```python
from build123d import *

# Parameters (mm, degrees)
SKETCH1_W           = 93.98
SKETCH1_H           = 66.04
SKETCH1_W_2         = 83.82
SKETCH1_H_2         = 55.88
BOSS_EXTRUDE1_DEPTH = 15.24
SKETCH3_W           = 83.82
SKETCH3_H           = 55.88
BOSS_EXTRUDE2_DEPTH = 7.62
BOSS_EXTRUDE3_DEPTH = 10
FILLET1_R           = 2.54
CUT_EXTRUDE1_DEPTH  = 16.24


with BuildPart() as part:
    # Sketch1 → Boss-Extrude1 (new body)
    with BuildSketch(Plane(origin=(0, 0, 0), x_dir=(1, 0, 0), z_dir=(0, 1, 0))):
        Rectangle(SKETCH1_W, SKETCH1_H)
        Rectangle(SKETCH1_W_2, SKETCH1_H_2, mode=Mode.SUBTRACT)
    extrude(amount=BOSS_EXTRUDE1_DEPTH)

    # Sketch3 → Boss-Extrude2 (add)
    with BuildSketch(Plane(origin=(0, 0, 0), x_dir=(1, 0, 0), z_dir=(0, 1, 0))):
        Rectangle(SKETCH3_W, SKETCH3_H)
    extrude(amount=BOSS_EXTRUDE2_DEPTH)

    # Sketch4 → Boss-Extrude3 (add)
    with BuildSketch(Plane.XZ):
        with BuildLine():
            Line((-30.48, 7.62), (30.48, 7.62))
            ThreePointArc((30.48, 7.62), (31.75, 6.35), (30.48, 5.08))
            Line((30.48, 5.08), (-30.48, 5.08))
            ThreePointArc((-30.48, 5.08), (-31.75, 6.35), (-30.48, 7.62))
        make_face()
    extrude(amount=BOSS_EXTRUDE3_DEPTH)

    # Fillet1
    fillet1_edges = [part.edges().sort_by_distance(p)[0] for p in [
        (46.99, 15.24, 0),
        (0, 15.24, -33.02),
        (-46.99, 15.24, 0),
        (0, 0, -33.02),
        (46.99, 0, 0),
        (0, 0, 33.02),
        (-46.99, 0, 0),
        (-46.99, 7.62, -33.02),
        (46.99, 7.62, -33.02),
        (46.99, 7.62, 33.02),
        (-46.99, 7.62, 33.02),
        (0, 15.24, 33.02),
    ]]
    fillet(fillet1_edges, radius=FILLET1_R)

    # Sketch5 → Cut-Extrude1 (cut, through all)
    with BuildSketch(Plane.XZ):
        with BuildLine():
            Line((38.1, 0), (8.720286281, 0))
            add(Edge.make_bspline(
                [(8.720286281, 0), (0.717932636, -10.320966423), (24.690327376, -11.221788079), (14.302617373, -24.27956655), (19.287221421, -25.4)],
                knots=[0, 0, 0, 0, 0.689243554, 1, 1, 1, 1], degree=3))
            Line((19.287221421, -25.4), (38.1, -25.4))
            Line((38.1, -25.4), (38.1, 0))
        make_face()
        with BuildLine():
            add(Edge.make_bspline(
                [(-38.1, -17.337980958), (-35.187970865, -6.837732589), (-22.396079464, -19.547216799), (-11.076568018, -5.424698839), (8.04848315, -15.407822573), (0.32989112, -20.213116903), (-0.131881687, -22.594944987), (-0.12685046, -22.796669294)],
                knots=[0, 0, 0, 0, 0.327916539, 0.565865574, 0.827054789, 0.928649045, 0.941908126, 0.941908126, 0.941908126, 0.941908126], degree=3))
            Line((-38.1, -17.337980958), (-38.1, -25.4))
            Line((-38.1, -25.4), (-2.666060814, -25.4))
            ThreePointArc((-2.666060814, -25.4), (-0.84775666, -24.633519101), (-0.12685046, -22.796669294))
        make_face()
        with BuildLine():
            ThreePointArc((-20.809664595, 23.563761473), (-23.399285475, 24.661043475), (-26.141098135, 24.03444358))
            ThreePointArc((-26.141098135, 24.03444358), (-32.141459521, 16.03667712), (-22.24223462, 14.631703292))
            ThreePointArc((-22.24223462, 14.631703292), (-20.680528135, 15.549204987), (-18.904626197, 15.192962357))
            ThreePointArc((-18.904626197, 15.192962357), (-17.075188661, 14.538079772), (-15.140614659, 14.720113645))
            ThreePointArc((-15.140614659, 14.720113645), (-13.518109108, 14.699820982), (-12.238965098, 13.701458994))
            ThreePointArc((-12.238965098, 13.701458994), (-9.256805246, 11.946815164), (-6.043815629, 13.230851799))
            ThreePointArc((-6.043815629, 13.230851799), (-4.644606266, 14.021459072), (-3.050933479, 13.813965102))
            ThreePointArc((-3.050933479, 13.813965102), (-0.202264641, 13.116417687), (2.681966092, 13.648112737))
            ThreePointArc((2.681966092, 13.648112737), (4.032557322, 13.814175625), (5.275046214, 13.259292838))
            ThreePointArc((5.275046214, 13.259292838), (7.732359851, 12.317746114), (10.257976284, 13.056773974))
            ThreePointArc((10.257976284, 13.056773974), (11.524940775, 13.507829697), (12.844614733, 13.248771918))
            ThreePointArc((12.844614733, 13.248771918), (15.999143067, 12.5855131), (19.076925277, 13.543749992))
            ThreePointArc((19.076925277, 13.543749992), (20.340690392, 13.925639815), (21.625421379, 13.621652327))
            ThreePointArc((21.625421379, 13.621652327), (23.29387293, 13.01462201), (25.066504565, 12.914654647))
            ThreePointArc((25.066504565, 12.914654647), (25.635512485, 12.901960546), (26.187409107, 12.762887643))
            ThreePointArc((26.187409107, 12.762887643), (32.302173237, 15.205977496), (30.433254549, 21.519943868))
            ThreePointArc((30.433254549, 21.519943868), (29.982257618, 21.867122384), (29.619886936, 22.306005788))
            ThreePointArc((29.619886936, 22.306005788), (26.018947716, 24.881341954), (21.625421379, 24.337240894))
            ThreePointArc((21.625421379, 24.337240894), (20.340690392, 24.033253406), (19.076925277, 24.415143229))
            ThreePointArc((19.076925277, 24.415143229), (13.537462145, 25.005428585), (9.633287177, 21.031575742))
            add(Edge.make_bspline(
                [(8.636564486, 20.482159427), (9.365510622, 20.380358696), (9.633287177, 21.031575742)],
                knots=[0, 0, 0, 1, 1, 1], degree=2))
            ThreePointArc((8.636564486, 20.482159427), (7.41195629, 21.075462315), (6.669321907, 22.215711291))
            ThreePointArc((6.669321907, 22.215711291), (-0.249726214, 27.097956484), (-6.802730996, 21.734406043))
            ThreePointArc((-6.802730996, 21.734406043), (-7.651745104, 20.369846866), (-9.149857761, 19.788034897))
            ThreePointArc((-9.149857761, 19.788034897), (-9.457684051, 19.760912808), (-9.762426275, 19.709679919))
            ThreePointArc((-9.762426275, 19.709679919), (-11.373542368, 19.902659169), (-12.539082341, 21.031575742))
            ThreePointArc((-12.539082341, 21.031575742), (-14.960654672, 23.176356644), (-18.19513891, 23.129352581))
            ThreePointArc((-18.19513891, 23.129352581), (-19.563553579, 22.978509725), (-20.809664595, 23.563761473))
        make_face()
    extrude(amount=-CUT_EXTRUDE1_DEPTH, mode=Mode.SUBTRACT)


solid = part.part
```
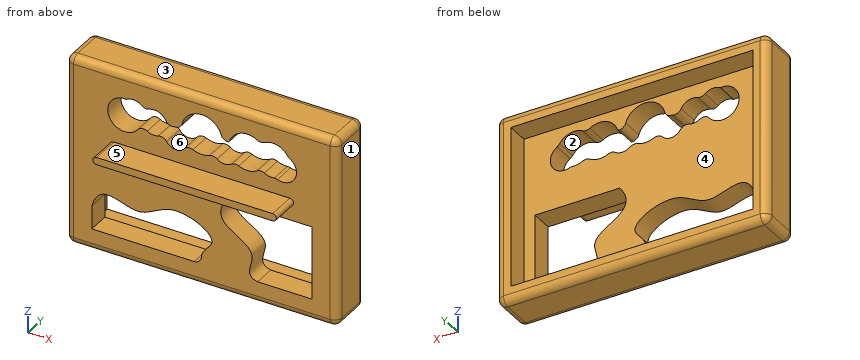
Work out the finished part from the listing and answer in its coordinate system (mm). Face numbers are marked on the shaded views. A direction names the side the tool comes from. Coordinates: 2 decimals unless noted, no trailing zeros. Write each loop counter-clockwise with the first axis right and the second up, starting at its lowest first coordinate (ties: lowest second). Pieces come first, ordered by that corner, then holes.
Q1. A cutting plane is placed at C-C, the plane z = 18. Give the vertices of the cut face in (x, y), then the cut area to 3 significant figures.
Q2. A cutting plane is placed at B-B, the plane y = 9.75. Give the vertices of the cut face in (x, z), then the cut area to 3 significant figures.
Q3. A cutting plane is placed at A-A, the plane z = 6.35. Give the vertices of the cut face in (x, y), then the cut area to 3 significant figures.
Q4. A cutting plane is placed at D-D, the plane x = -16.5. State how many separate pieces and enclosed holes the cut face has, then the cut area to 3 significant figures.
Q5. Each of these flat-tipped pins is pushed along its axis until it touches: pin 1 Ø1.5 at (x, y) = (8, -7) entering from +Z; pin 2 Ø11 at (x, y) = (11.5, -4.5) entering from +Z; pin 3 Ø8 at (x, z) = (1, -3.5) entering from +Y; pin 4 Ø1.5 at (y, z) = (-2.5, -9.5) entering from +X (3 decimals). Where does it stop, or does it pass through?
Q6. Determine the mould class of the marked faces 1, 2 and 3 for opening direction Z: released by +Z, released by -Z, zero draft, split by the parting line, or undercut.
Q7. Which of the six approach directions +Z, -Z, +X, -X, +Y, -Y give full straight-line access (tool end or side, diameter ignored) to the marked faces 4, 5 and 6?
Q8. Find the intervals of material crossed by line 1 (X direction, y = 11.5, z = -2); line 2 (Z direction, x = -31, y = 9); line 3 (Z direction, x = 11.5, y = 2), in increasing order.
Findings below:
1. outline: (-46.99, 2.54) arc R2.54 ccw to (-44.45, 0) - (-32.58, 0) - (-32.58, 7.62) - (-41.91, 7.62) - (-41.91, 15.24) - (-44.45, 15.24) arc R2.54 ccw to (-46.99, 12.7) - close; (32.75, 0) - (44.45, 0) arc R2.54 ccw to (46.99, 2.54) - (46.99, 12.7) arc R2.54 ccw to (44.45, 15.24) - (41.91, 15.24) - (41.91, 7.62) - (32.75, 7.62) - close
1. area: 290 mm2
2. outline: (-46.99, -30.48) arc R2.54 ccw to (-44.45, -33.02) - (44.45, -33.02) arc R2.54 ccw to (46.99, -30.48) - (46.99, 30.48) arc R2.54 ccw to (44.45, 33.02) - (-44.45, 33.02) arc R2.54 ccw to (-46.99, 30.48) - close; hole (-41.91, -27.94) - (41.91, -27.94) - (41.91, 27.94) - (-41.91, 27.94) - close
2. area: 1,520 mm2
3. outline: (-46.99, 2.54) arc R2.54 ccw to (-44.45, 0) - (-31.75, 0) - (-31.75, -10) - (31.75, -10) - (31.75, 0) - (44.45, 0) arc R2.54 ccw to (46.99, 2.54) - (46.99, 12.7) arc R2.54 ccw to (44.45, 15.24) - (41.91, 15.24) - (41.91, 7.62) - (-41.91, 7.62) - (-41.91, 15.24) - (-44.45, 15.24) arc R2.54 ccw to (-46.99, 12.7) - close
3. area: 1,420 mm2
4. separate pieces: 3
4. enclosed holes: 0
4. area: 431 mm2
5. pin 1: stops at z = 7.62
5. pin 2: stops at z = 32.5
5. pin 3: stops at y = 7.62
5. pin 4: passes through
6. face 1: zero draft
6. face 2: undercut
6. face 3: released by +Z
7. face 4: +Y
7. face 5: +Z, +X, -X, -Y
7. face 6: +Y, -Y
8. line 1: x = -46.99 to -41.91, 41.91 to 46.99
8. line 2: z = -33.02 to -27.94, 27.94 to 33.02
8. line 3: z = -32.96 to -11.14, 0 to 13.51, 23.81 to 32.96
